```python
from build123d import *

# Parameters (mm, degrees)
SKETCH_W        = 129
SKETCH_H        = 130
PAD_DEPTH       = 1.5
SKETCH001_R     = 13.85
PAD001_DEPTH    = 12.5
SKETCH002_R     = 12.3
POCKET_DEPTH    = 12.5
SKETCH003_W     = 3
SKETCH003_H     = 3.5
POCKET001_DEPTH = 12.5
SKETCH004_W     = 8
SKETCH004_H     = 27.2
PAD002_DEPTH    = 26
SKETCH005_R     = 2
PAD003_DEPTH    = 2
SKETCH006_W     = 5
SKETCH006_H     = 14
PAD004_DEPTH    = 51.5
SKETCH007_R     = 4
POCKET002_DEPTH = 5


with BuildPart() as part:
    # Sketch → Pad (new body)
    with BuildSketch(Plane.XY):
        Rectangle(SKETCH_W, SKETCH_H)
    extrude(amount=PAD_DEPTH)

    # Sketch001 (on Face6 of Pad) → Pad001 (join)
    with BuildSketch(Plane.XY.offset(1.5)):
        with Locations((16, 0)):
            Circle(SKETCH001_R)
    extrude(amount=PAD001_DEPTH)

    # Sketch002 (on Face8 of Pad001) → Pocket (cut)
    with BuildSketch(Plane.XY.offset(14)):
        with Locations((16, 0)):
            Circle(SKETCH002_R)
    extrude(amount=-POCKET_DEPTH, mode=Mode.SUBTRACT)

    # Sketch003 (on Face8 of Pocket) → Pocket001 (cut)
    with BuildSketch(Plane.XY.offset(14)):
        with Locations((16, -12.75)):
            Rectangle(SKETCH003_W, SKETCH003_H)
    extrude(amount=-POCKET001_DEPTH, mode=Mode.SUBTRACT)

    # Sketch004 (on Face5 of Pocket001) → Pad002 (join)
    with BuildSketch(Plane.XY.offset(1.5)):
        with Locations((35, 0)):
            Rectangle(SKETCH004_W, SKETCH004_H)
        with Locations((-35, 0)):
            Rectangle(SKETCH004_W, SKETCH004_H)
    extrude(amount=PAD002_DEPTH)

    # Sketch005 (on Face23 of Pad002) → Pad003 (join)
    with BuildSketch(Plane.XY.offset(27.5)):
        with Locations((35, 7.5)):
            Circle(SKETCH005_R)
        with Locations((35, -7.5)):
            Circle(SKETCH005_R)
        with Locations((-35, 7.5)):
            Circle(SKETCH005_R)
        with Locations((-35, -7.5)):
            Circle(SKETCH005_R)
    extrude(amount=PAD003_DEPTH)

    # Sketch006 (on Face5 of Pad003) → Pad004 (join)
    with BuildSketch(Plane.XY.offset(1.5)):
        with Locations((23.75, 51.75)):
            Rectangle(SKETCH006_W, SKETCH006_H)
    extrude(amount=PAD004_DEPTH)

    # Sketch007 (on Face15 of Pad004) → Pocket002 (cut)
    with BuildSketch(Plane.YZ.offset(26.25)):
        with Locations((51.511597, 45.262314)):
            Circle(SKETCH007_R)
    extrude(amount=-POCKET002_DEPTH, mode=Mode.SUBTRACT)


solid = part.part
```
Work out the finished part from the listing and answer in its coordinate system (mm). A direction names the side the tool comes from. Round coordinates to 2 decimals unless told otherwise and drop trailing zeros. Write each loop counter-clockwise with the first axis right and the second up, starting at its lowest first coordinate (ties: lowest second). Pieces come first, ordered by that corner, then holes. Notation, with made-up numbers: (20, 64) -> (64, 64) arc R17 ccw to (64, 97) -> close; hole circle Ø5 at (52, 29.25). An arc over 180 degrees is marked (long way). Write each question's results on one line, items separated by ' | '.
1) Flat-ended cylindrical pins translate along their axes: pin 1 (6.5 mm diameter, centred on x = 34.5, y = 1.5, fed in from +Z); pin 2 (21 mm diameter, centred on y = -0.5, z = 13.5, fed in from +X); pin 3 (4.5 mm diameter, centred on x = 34.5, y = -8, fed in from +Z); pin 4 (12 mm diameter, centred on y = 33.5, z = 9, fed in from -X). Find the tip coordinate at first contact, or state that the pin passes through.
Findings:
pin 1: stops at z = 27.5 | pin 2: stops at x = 39 | pin 3: stops at z = 29.5 | pin 4: passes through
2) The part is cut by section A-A (x = -35). Write down the section's boundary in (y, z), and give its area (3 significant figures).
Findings:
outline: (-65, 0) -> (65, 0) -> (65, 1.5) -> (13.6, 1.5) -> (13.6, 27.5) -> (9.5, 27.5) -> (9.5, 29.5) -> (5.5, 29.5) -> (5.5, 27.5) -> (-5.5, 27.5) -> (-5.5, 29.5) -> (-9.5, 29.5) -> (-9.5, 27.5) -> (-13.6, 27.5) -> (-13.6, 1.5) -> (-65, 1.5) -> close | area: 918 mm²
3) The part is cut by section C-C (y = 0). Write down the section's boundary in (x, z), and give its area (3 significant figures).
Findings:
outline: (-64.5, 0) -> (64.5, 0) -> (64.5, 1.5) -> (39, 1.5) -> (39, 27.5) -> (31, 27.5) -> (31, 1.5) -> (29.85, 1.5) -> (29.85, 14) -> (28.3, 14) -> (28.3, 1.5) -> (3.7, 1.5) -> (3.7, 14) -> (2.15, 14) -> (2.15, 1.5) -> (-31, 1.5) -> (-31, 27.5) -> (-39, 27.5) -> (-39, 1.5) -> (-64.5, 1.5) -> close | area: 648 mm²
4) Consider line 1 along X through (y, z) = (0, 8); line 2 along X through (y, z) = (6.5, 21); line 3 along Y through (x, z) = (19, 4). Determine where each line is inside the solid, lowest interval first. Write a range as [from, to].
Findings:
line 1: x = [-39, -31], [2.15, 3.7], [28.3, 29.85], [31, 39] | line 2: x = [-39, -31], [31, 39] | line 3: y = [-13.52, -11.93], [11.93, 13.52]
5) The part is cut by section D-D (z = 43). Write down the section's boundary in (x, y).
Findings:
outline: (21.25, 44.75) -> (26.25, 44.75) -> (26.25, 48.21) -> (21.25, 48.21) -> close; (21.25, 54.81) -> (26.25, 54.81) -> (26.25, 58.75) -> (21.25, 58.75) -> close
6) For a pull along X with two mould halves and no side action, classify faces 1 (the flat face through (35, -13.6, 14)), 2 (the cylindrical face through (36.908, 8.101, 28.486)) as +X half, -X half, draft (parallel to the pull), parting line (faces both ways), or undercut.
Findings:
face 1: draft | face 2: undercut
7) The part is cut by section B-B (z = 6.5). Write down the section's boundary in (x, y), and give its area (3 significant figures).
Findings:
outline: (-39, -13.6) -> (-31, -13.6) -> (-31, 13.6) -> (-39, 13.6) -> close; (14.5, -13.77) -> (14.5, -12.21) arc R12.3 cw (long way) to (17.5, -12.21) -> (17.5, -13.77) arc R13.85 ccw (long way) to start; (21.25, 44.75) -> (26.25, 44.75) -> (26.25, 58.75) -> (21.25, 58.75) -> close; (31, -13.6) -> (39, -13.6) -> (39, 13.6) -> (31, 13.6) -> close | area: 628 mm²
8) Which of the six approach directions +Z, -Z, +X, -X, +Y, -Y give full straight-line access (tool end or side, diameter ignored) to faces 3 (the flat face through (-31, 0, 14)), 4 (the flat face through (7.7, 9.3, 14)), 5 (the flat face through (35, 0, 27.5)), 6 (the flat face through (-35, -13.6, 14))?
Findings:
face 3: +Z, +Y, -Y | face 4: +Z, -Y | face 5: +Z | face 6: +Z, -X, -Y
